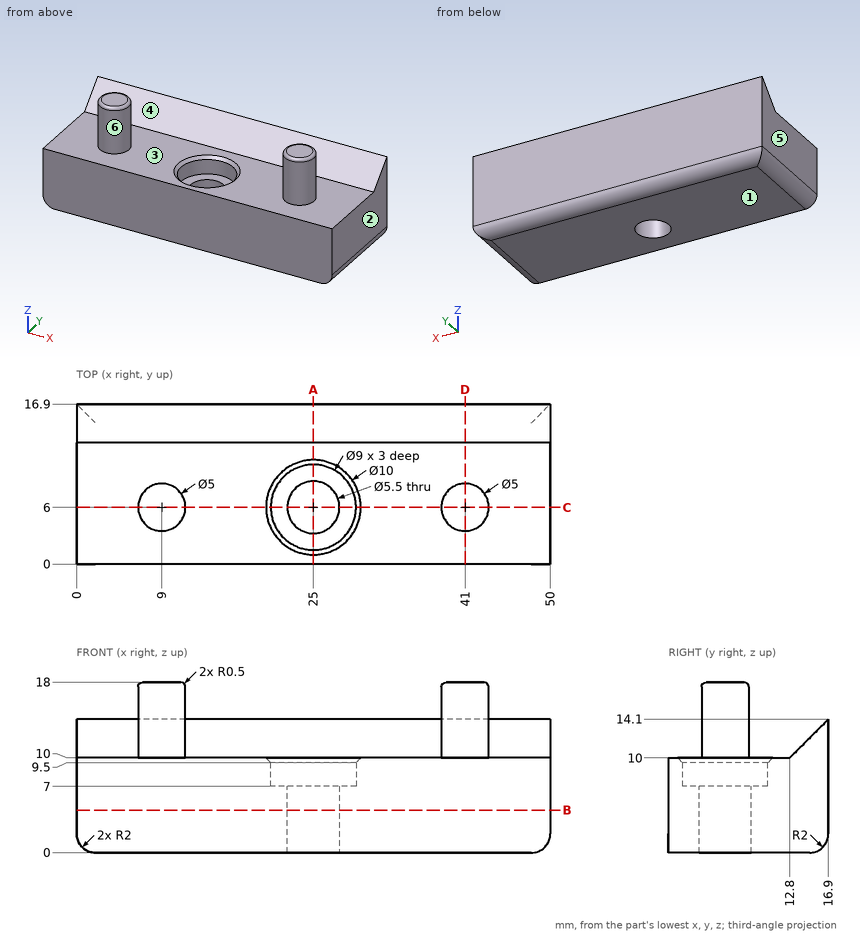
Design review of the part shown in the three views and the two pictorial views. Dimensions are in mm from the part's minimum x, y and z. A direction names the side the tool comes from. Coordinates: 2 decimals unless noted, no trailing zeros. Order: outer loops, then holes, each group sorted by start corner. A loop starts at its lowest first (then second) coordinate and runs counter-clockwise, first axis right, second up. Notation, with made-up numbers: (86.5, 2) -> (143.5, 2) arc R16 cw to (143.5, 23) -> close; hole circle Ø3 at (24.5, -5). An arc over 180 degrees is marked (long way). Use one line per item in the form item = value. Start each with the question number.
(1) The part is to be moulded in two halves that separate along X. For the marked faces 1, 2 and 3, say which applies: +X half, -X half, draft (parallel to the pull), parting line (faces both ways), or undercut.
(2) For probe 1 along Y at (x, z) = (25, 7.9); probe 2 along Y at (x, z) = (25, 3.25); probe 3 along X at (y, z) = (6.25, 3.5), list the stretches that pass through material, from the lowest coordinate up.
(3) Add section D-D on x = 41. State the section outline as (y, z) points.
(4) Add section B-B on z = 4.5. State the section outline as (x, y) points, plus the area to 3 significant figures.
(5) Insertion check: pin 1 (3.5 mm diameter, centred on x = 25, y = 6, fed in from +Z); pin 2 (2 mm diameter, centred on x = 21.5, y = 10, fed in from +Z); pin 3 (2.5 mm diameter, centred on x = 23.5, y = 4, fed in from +Z); pin 4 (1 mm diameter, centred on y = 5.5, z = 14.5, fed in from -X). Each pin has a flat end and moves straight along its axis. Give the tip position at first contact, or say it passes through.
(6) Add section C-C on y = 6. State the section outline as (x, z) points.
(7) Add section A-A on x = 25. State the section outline as (y, z) points.
(8) For the marked faces 4, 5 and 6, list the 3-axis set-ups (+Z, -Z, +X, -X, +Y, -Y) from which the entire face can be reached by the end or side of a thin tool; tool diameter is ignored.
Answer block:
q1.face_1 = draft
q1.face_2 = +X half
q1.face_3 = undercut
q2.probe_1 = 0 to 1.5, 10.5 to 16.9
q2.probe_2 = 0 to 3.25, 8.75 to 16.9
q2.probe_3 = 0 to 22.26, 27.74 to 50
q3.outline = (0, 0) -> (14.9, 0) arc R2 ccw to (16.9, 2) -> (16.9, 14.1) -> (12.8, 10) -> (8.5, 10) -> (8.5, 17.5) arc R0.5 ccw to (8, 18) -> (4, 18) arc R0.5 ccw to (3.5, 17.5) -> (3.5, 10) -> (0, 10) -> close
q4.outline = (0, 0) -> (50, 0) -> (50, 16.9) -> (0, 16.9) -> close; hole circle Ø5.5 at (25, 6)
q4.area = 821 mm²
q5.pin_1 = through
q5.pin_2 = 10
q5.pin_3 = 7
q5.pin_4 = 6.5
q6.outline = (0, 2) arc R2 ccw to (2, 0) -> (22.25, 0) -> (22.25, 7) -> (20.5, 7) -> (20.5, 9.5) -> (20, 10) -> (11.5, 10) -> (11.5, 17.5) arc R0.5 ccw to (11, 18) -> (7, 18) arc R0.5 ccw to (6.5, 17.5) -> (6.5, 10) -> (0, 10) -> close; (27.75, 0) -> (48, 0) arc R2 ccw to (50, 2) -> (50, 10) -> (43.5, 10) -> (43.5, 17.5) arc R0.5 ccw to (43, 18) -> (39, 18) arc R0.5 ccw to (38.5, 17.5) -> (38.5, 10) -> (30, 10) -> (29.5, 9.5) -> (29.5, 7) -> (27.75, 7) -> close
q7.outline = (0, 0) -> (3.25, 0) -> (3.25, 7) -> (1.5, 7) -> (1.5, 9.5) -> (1, 10) -> (0, 10) -> close; (8.75, 0) -> (14.9, 0) arc R2 ccw to (16.9, 2) -> (16.9, 14.1) -> (12.8, 10) -> (11, 10) -> (10.5, 9.5) -> (10.5, 7) -> (8.75, 7) -> close
q8.face_4 = +Z, +X, -X
q8.face_5 = +Z, -Z, -X, +Y, -Y
q8.face_6 = +Z
